Input: part model. Units: mm. Frame: model coordinates. A direction names the side the tool comes from. Give positions to 0.01 mm unless a question says otherwise; leave off trailing zeros. Loops run counter-clockwise (first coordinate to the right, second up) from the corner with the lowest first, then second, coordinate; pieces in that order, holes last.
Autodesk Inventor part; units mm, degrees
ref_plane "YZ Plane" through (0, 0, 0) normal (1, 0, 0) x (0, 1, 0)
ref_plane "XZ Plane" through (0, 0, 0) normal (0, 1, 0) x (-1, 0, 0)
ref_plane "XY Plane" through (0, 0, 0) normal (0, 0, 1) x (1, 0, 0)
sketch "Sketch1" plane through (0, 0, 0) normal (0, 1, 0) x (-1, 0, 0)
  circle A0 centre (32.5, 0) radius 12
  circle A1 centre (-32.5, 0) radius 12
  line L0 (32.5, 12) -> (-32.5, 12)
  line L1 (32.5, -12) -> (-32.5, -12)
  circle A2 centre (32.5, 0) radius 3.75
  circle A3 centre (-32.5, 0) radius 3.75
  line L2 (62.3, 0) -> (-62.3, 0)
  circle A4 centre (32.5, -7) radius 1
  circle A5 centre (32.5, 7) radius 1
  circle A6 centre (-32.5, -7) radius 1
  circle A7 centre (-32.5, 7) radius 1
  line L3 (2.5, -5) -> (-2.5, -5)
  line L4 (-2.5, -5) -> (-2.5, 5)
  line L5 (-2.5, 5) -> (2.5, 5)
  line L6 (2.5, 5) -> (2.5, -5)
  point P0 (0, 0)
  point P1 (0, 12)
  point P2 (2.5, 0)
  point P3 (0, -5)
  dimension "d5" = 65
  dimension "d6" = 24
  dimension "d7" = 7.5
  dimension "d17" = 2
  dimension "d18" = 7
  dimension "d19" = 7
  dimension "d25" = 5
  dimension "d26" = 10
extrude "Extrusion7" add sketch "Sketch1" along normal blind 5 contours L2 A2 A0 | A0 L2 A2 | A0 L2 L6 L5 L4 A1 L0 | L1 A1 L2 L4 L3 L6 A0 | A1 L2 A3 | A1 L2 A3
sketch "Sketch4" plane through (0, 5, 0) normal (0, 1, 0) x (1, 0, 0)
  circle A0 centre (-32.5, -7) radius 2
  circle A1 centre (-32.5, 7) radius 2
  circle A2 centre (32.5, -7) radius 2
  circle A3 centre (32.5, 7) radius 2
  circle A4 centre (-32.5, -7) radius 1
  circle A5 centre (-32.5, 7) radius 1
  circle A6 centre (32.5, -7) radius 1
  circle A7 centre (32.5, 7) radius 1
  point P0 (0, 0)
  dimension "d29" = 4
extrude "Extrusion8" cut sketch "Sketch4" against normal blind 1
equation "\"d6\" = sa_diameter"
equation "\"d25\" = b_mat_thickness"
equation "\"d27\" = b_mat_thickness"
properties part number "Middle_leg_a"
(1) Reachability of faces 1 (the flat face through (-31.6, 4, -6.1)), 2 (the flat face through (0, 2, 5)), 3 (the flat face through (1, 5, 6)) from +Z, -Z, +X, -X, +Y, -Y: full face, straight path, thin tool, end or side. Return the list, or none.
Values follow:
face 1: +Y
face 2: +Y, -Y
face 3: +Z, -Z, +X, -X, +Y
(2) Cut plane D-D (x = -1). Return the cut outline in (y, z), and give its area (3 significant figures).
Values follow:
outline: (0, -12) - (5, -12) - (5, -5) - (0, -5) - close; (0, 5) - (5, 5) - (5, 12) - (0, 12) - close
area: 70.0 mm2
(3) Mould query, pull axis X, two halves, no side actions, for faces 4 (the cylindrical face through (-44.497, 2.465, 0.264)), 5 (the cylindrical face through (33.237, 1.972, -7.676)), 6 (the cylindrical face through (44.497, 2.465, -0.264)), 7 (the flat face through (1, 0, 6)). Classes: +X half, -X half, draft (parallel to the pull), parting line (faces both ways), or undercut.
Values follow:
face 4: -X half
face 5: undercut
face 6: +X half
face 7: draft
(4) Cut plane B-B (z = 0). Return the cut outline in (x, y).
Values follow:
outline: (-44.5, 0) - (-36.25, 0) - (-36.25, 5) - (-44.5, 5) - close; (-28.75, 0) - (-2.5, 0) - (-2.5, 5) - (-28.75, 5) - close; (2.5, 0) - (28.75, 0) - (28.75, 5) - (2.5, 5) - close; (36.25, 0) - (44.5, 0) - (44.5, 5) - (36.25, 5) - close
(5) Cut plane C-C (y = 1.25). Return the cut outline in (x, z), and give its area (3 significant figures).
Values follow:
outline: (-32.5, -12) - (32.5, -12) arc R12 ccw to (32.5, 12) - (-32.5, 12) arc R12 ccw to start; hole circle Ø7.5 at (-32.5, 0); hole circle Ø2 at (-32.5, -7); hole circle Ø2 at (-32.5, 7); hole (-2.5, -5) - (2.5, -5) - (2.5, 5) - (-2.5, 5) - close; hole circle Ø7.5 at (32.5, 0); hole circle Ø2 at (32.5, -7); hole circle Ø2 at (32.5, 7)
area: 1,860 mm2
(6) Ray query, probe 1 along Z at (x, y) = (32.5, 2.3); probe 2 along X at (y, z) = (3.85, 0); probe 3 along X at (y, z) = (4.1, 3). Return the intervals inside material, ascending.
Values follow:
probe 1: z = -12 to -8, -6 to -3.75, 3.75 to 6, 8 to 12
probe 2: x = -44.5 to -36.25, -28.75 to -2.5, 2.5 to 28.75, 36.25 to 44.5
probe 3: x = -44.12 to -34.75, -30.25 to -2.5, 2.5 to 30.25, 34.75 to 44.12
(7) Pin query (flat end, axial travel): pin 1 Ø2 at (x, z) = (-32.5, -7.5) entering from +Y; pin 2 Ø1 at (y, z) = (3.5, 6.5) entering from -X; pin 3 Ø3 at (y, z) = (2.5, -2.5) entering from -X. Return the tip coordinate at first contact, or that it passes through.
Values follow:
pin 1: stops at y = 4
pin 2: stops at x = -42.89
pin 3: stops at x = -44.46
(8) Cut plane A-A (x = 29.5). Return the cut outline in (y, z).
Values follow:
outline: (0, -12) - (5, -12) - (5, -2.25) - (0, -2.25) - close; (0, 2.25) - (5, 2.25) - (5, 12) - (0, 12) - close
